Here's how the part is built. I have some questions about the finished solid (model axes, mm). Round coordinates to 2 decimals unless told otherwise and drop trailing zeros. Write each loop counter-clockwise with the first axis right and the second up, starting at its lowest first coordinate (ties: lowest second). Pieces come first, ordered by that corner, then holes. Notation, with made-up numbers: (45, 72.5) -> (77, 72.5) arc R23 ccw to (77, 104.5) -> close; hole circle Ø1 at (-28.75, 39.25). An arc over 180 degrees is marked (long way). Answer in a Markdown table with one row per item. Add a question column.
from build123d import *

# Parameters (mm, degrees)
BOSS_EXTRUDE1_DEPTH = 12.77
SKETCH2_W           = 529.42
SKETCH2_H           = 36.4
CUT_EXTRUDE1_DEPTH  = 1
SKETCH3_R           = 2.5
SKETCH3_W           = 34.32
SKETCH3_H           = 14.88
BOSS_EXTRUDE2_DEPTH = 1.25


with BuildPart() as part:
    # Sketch1 → Boss-Extrude1 (new body)
    with BuildSketch(Plane.XY):
        with BuildLine():
            Line((-269.21, 27.35), (269.21, 27.35))
            ThreePointArc((269.21, 27.35), (270.624213562, 26.764213562), (271.21, 25.35))
            Line((271.21, 25.35), (271.21, -25.35))
            ThreePointArc((271.21, -25.35), (270.624213562, -26.764213562), (269.21, -27.35))
            Line((269.21, -27.35), (-269.21, -27.35))
            ThreePointArc((-269.21, -27.35), (-270.624213562, -26.764213562), (-271.21, -25.35))
            Line((-271.21, -25.35), (-271.21, 25.35))
            ThreePointArc((-271.21, 25.35), (-270.624213562, 26.764213562), (-269.21, 27.35))
        make_face()
    extrude(amount=BOSS_EXTRUDE1_DEPTH)

    # Sketch2 → Cut-Extrude1 (cut)
    with BuildSketch(Plane.XY.offset(12.77)):
        with Locations((0, -2.67)):
            Rectangle(SKETCH2_W, SKETCH2_H)
    extrude(amount=-CUT_EXTRUDE1_DEPTH, mode=Mode.SUBTRACT)

    # Sketch3 → Boss-Extrude2 (add)
    with BuildSketch(Plane(origin=(0, 0, 0), x_dir=(-1, 0, 0), z_dir=(0, 0, -1))):
        with Locations((-253.41, 4.02)):
            Circle(SKETCH3_R)
        with Locations((-253.41, -10.06)):
            Circle(SKETCH3_R)
        with Locations((-113, -10.06)):
            Circle(SKETCH3_R)
        with Locations(Location((113, -10.06, 0), (0, 0, 180))):
            Circle(SKETCH3_R)
        with Locations(Location((253.41, -10.06, 0), (0, 0, 180))):
            Circle(SKETCH3_R)
        with Locations(Location((253.41, 4.02, 0), (0, 0, 180))):
            Circle(SKETCH3_R)
        with Locations((0, -19.91)):
            Rectangle(SKETCH3_W, SKETCH3_H)
    extrude(amount=BOSS_EXTRUDE2_DEPTH)


solid = part.part
Item 1: I need wall thicknesses on line 1 along X through (y, z) = (-17, 12); line 2 along Z through (x, y) = (-75.5, 8.5); line 3 along Z through (x, y) = (132.5, -25). Which ranges of each line are inside material? Lowest first, please. Write a range as from..to.
Item 2: If we section it at B-B on x = 9.5: Please give me the cut outline in (y, z).
Item 3: If we mould it in two halves opening along X, with no side actions, what happens to faces 1 (the flat face through (-4, 27.35, 6)), 2 (the flat face through (-4, -2, 11.77)), 3 (the flat face through (-271.21, 0, 6))? For each: pulls with the +X half, pulls with the -X half, needs draft (parallel to the pull), parting line crosses it, or undercut.
Item 4: For P1, Ø1.4, axis at x = 8.5, z = -1, coming from the +Y side; P2, Ø0.6, axis at y = -21, z = -0.5, coming from the -X side; P3, Ø10, axis at x = 154, y = 0, coming from the +Z side, each with a flat end and sliding along its axis, tell me the tip position at first contact or that it passes through.
Item 5: If we section it at A-A on x = -232.5: Please give me the cut outline in (y, z).
Results list:
| question | item | result |
|---|---|---|
| 1 | line 1 | -271.21..-264.71, 264.71..271.21 |
| 1 | line 2 | 0..11.77 |
| 1 | line 3 | 0..12.77 |
| 2 | outline | (-27.35, -1.25) -> (-12.47, -1.25) -> (-12.47, 0) -> (27.35, 0) -> (27.35, 12.77) -> (15.53, 12.77) -> (15.53, 11.77) -> (-20.87, 11.77) -> (-20.87, 12.77) -> (-27.35, 12.77) -> close |
| 3 | face 1 | needs draft |
| 3 | face 2 | undercut |
| 3 | face 3 | pulls with the -X half |
| 4 | P1 | y = -12.47 |
| 4 | P2 | x = -17.16 |
| 4 | P3 | z = 11.77 |
| 5 | outline | (-27.35, 0) -> (27.35, 0) -> (27.35, 12.77) -> (15.53, 12.77) -> (15.53, 11.77) -> (-20.87, 11.77) -> (-20.87, 12.77) -> (-27.35, 12.77) -> close |
